```python
from build123d import *

# Parameters (mm, degrees)
SKETCH1_W           = 10.3
SKETCH1_H           = 10.3
BOSS_EXTRUDE1_DEPTH = 0.5
SKETCH2_R           = 5
BOSS_EXTRUDE2_DEPTH = 9.5
CHAMFER1_SIZE       = 1.5
FILLET1_R           = 0.5


with BuildPart() as part:
    # Sketch1 → Boss-Extrude1 (new body)
    with BuildSketch(Plane(origin=(0, 0, 0), x_dir=(1, 0, 0), z_dir=(0, 1, 0))):
        Rectangle(SKETCH1_W, SKETCH1_H)
    extrude(amount=BOSS_EXTRUDE1_DEPTH)

    # Sketch2 → Boss-Extrude2 (add)
    with BuildSketch(Plane(origin=(0, 0.5, 0), x_dir=(1, 0, 0), z_dir=(0, 1, 0))):
        with Locations(Location((0, 0, 0), (0, 0, 270))):
            Circle(SKETCH2_R)
    extrude(amount=BOSS_EXTRUDE2_DEPTH)

    # Chamfer1
    chamfer1_edges = [part.edges().sort_by_distance(p)[0] for p in [
        (5.15, 0.25, 5.15),
        (5.15, 0.25, -5.15),
    ]]
    chamfer(chamfer1_edges, length=CHAMFER1_SIZE)

    # Fillet1
    fillet1_edges = [part.edges().sort_by_distance(p)[0] for p in [
        (0, 10, -5),
    ]]
    fillet(fillet1_edges, radius=FILLET1_R)


solid = part.part
```
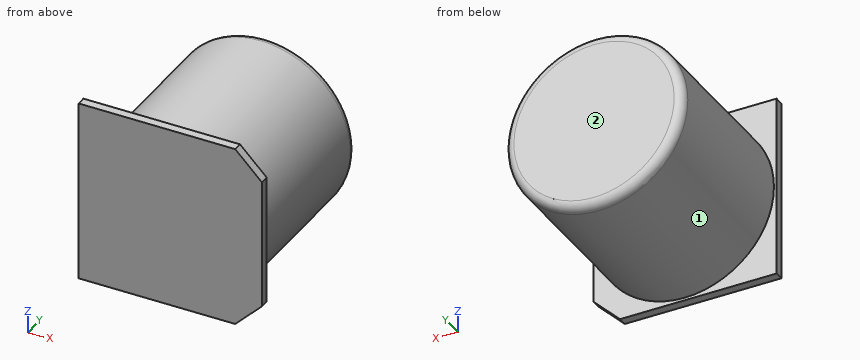
Here's how the part is built. I have some questions about the finished solid (model axes, mm). Face numbers are marked on the shaded views. A direction names the side the tool comes from. Round coordinates to 2 decimals unless told otherwise and drop trailing zeros. Order: outer loops, then holes, each group sorted by start corner. A loop starts at its lowest first (then second) coordinate and runs counter-clockwise, first axis right, second up. Notation, with made-up numbers: M 37,-26 L 85,-26 A7 ccw 85,-22 Z; hole C 41,48.25 d3. An arc over 180 degrees is marked long. Use CSV: the item, a comma, the result in double quotes.
1) I want a section at B-B (z = 0). List the corners of the cut face in (x, y) for me, then the cut area to 3 significant figures.
Taken from the geometry:
outline,"M -5.15,0 L 5.15,0 L 5.15,0.5 L 5,0.5 L 5,9.5 A0.5 ccw 4.5,10 L -4.5,10 A0.5 ccw -5,9.5 L -5,0.5 L -5.15,0.5 Z"
area,"100 mm^2"
2) On a 3-axis mill with a long thin cutter (end or side, diameter ignored), from which of +Z, -Z, +X, -X, +Y, -Y can I reach the whole of each face in a straight line? I mean the marked faces 1 and 2. Say none if no direction works.
Taken from the geometry:
face 1,"+Y"
face 2,"+Z, -Z, +X, -X, +Y"
3) I want a section at C-C (y = 6.5). List the corners of the cut face in (x, z) for me, then the cut area to 3 significant figures.
Taken from the geometry:
outline,"C 0,0 d10"
area,"78.5 mm^2"
4) I need wall thicknesses on line 1 along Y through (x, z) = (4, 3.5); line 2 along X through (y, z) = (3.25, 1.5); line 3 along X through (y, z) = (2.5, -4). Which ranges of each line are inside material? Lowest first, please. Write a range as [from, to].
Taken from the geometry:
line 1,"[0, 0.5]"
line 2,"[-4.77, 4.77]"
line 3,"[-3, 3]"
5) I'm going to push flat-ended pins straight in: P1, Ø6, axis at y = 6.5, z = 1, coming from the -X side; P2, Ø1, axis at y = 3.5, z = 3.5, coming from the -X side; P3, Ø1.5, axis at x = 4, y = 6, coming from the -Z side. Where does each tip first touch, or does it pass through?
Taken from the geometry:
P1,"x = -5"
P2,"x = -4"
P3,"z = -3.8"
6) I want a section at A-A (x = 0). List the corners of the cut face in (y, z) for me.
Taken from the geometry:
outline,"M 0,-5.15 L 0.5,-5.15 L 0.5,-5 L 9.5,-5 A0.5 ccw 10,-4.5 L 10,4.5 A0.5 ccw 9.5,5 L 0.5,5 L 0.5,5.15 L 0,5.15 Z"
